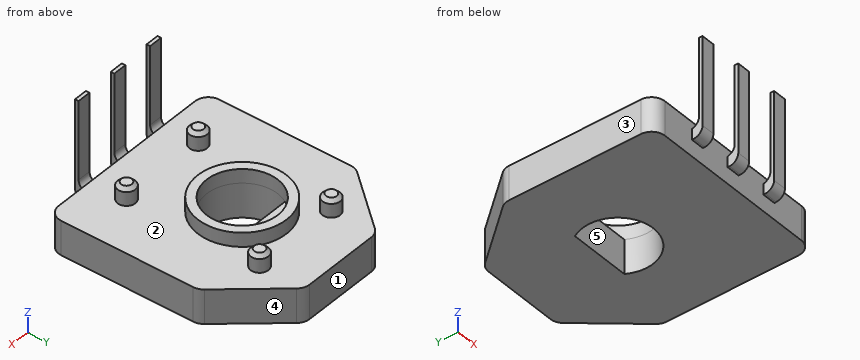
from build123d import *
from build123d.topology import SkipClean

# Parameters (mm, degrees)
BOSS_EXTRUDE1_DEPTH      = 1.93
SKETCH2_R                = 2.5
SKETCH2_R_2              = 2
BOSS_EXTRUDE2_DEPTH      = 0.79
BOSS_EXTRUDE3_DEPTH      = 4.5
BOSS_EXTRUDE3_DEPTH_BACK = 1
SKETCH3_W                = 0.76
SKETCH3_H                = 0.6
FILLET2_R                = 0.75
SKETCH4_W                = 5.74
SKETCH4_H                = 0.4
CUT_EXTRUDE1_DEPTH       = 4.9
FILLET1_R                = 0.5
SKETCH5_R                = 0.5
BOSS_EXTRUDE4_DEPTH      = 0.97
CHAMFER1_SIZE            = 0.2


with BuildPart() as part:
    # Sketch1 → Boss-Extrude1 (new body)
    with BuildSketch(Plane.XY):
        Polygon((5.5, 0), (5.5, -6.5), (-5.5, -6.5), (-5.5, 0), (-5.5, 1.96), (-2.49602332, 5.54), (2.49602332, 5.54), (5.5, 1.96), align=None)
        with BuildLine():
            Line((-1.718566554, 1.023), (1.718566554, 1.023))
            ThreePointArc((1.718566554, 1.023), (0, -2), (-1.718566554, 1.023))
        make_face(mode=Mode.SUBTRACT)
    extrude(amount=BOSS_EXTRUDE1_DEPTH)

    # Sketch2 → Boss-Extrude2 (add)
    with SkipClean():  # the faces are left unmerged after this step: merging them gives an invalid solid
        with BuildSketch(Plane.XY.offset(1.93)):
            with Locations(Location((0, 0, 0), (0, 0, 180))):
                Circle(SKETCH2_R)
            with Locations(Location((0, 0, 0), (0, 0, 149.236204264))):
                Circle(SKETCH2_R_2, mode=Mode.SUBTRACT)
        extrude(amount=BOSS_EXTRUDE2_DEPTH)

    # Sketch3 → Boss-Extrude3 (add, two sides: drawn at the far end of the back side and taken through both)
    with SkipClean():  # the faces are left unmerged after this step: merging them gives an invalid solid
        with BuildSketch(Plane.XY.offset(1.93).offset(-BOSS_EXTRUDE3_DEPTH_BACK)):
            with Locations((0, -6.8)):
                Rectangle(SKETCH3_W, SKETCH3_H)
            with Locations((2.49, -6.8)):
                Rectangle(SKETCH3_W, SKETCH3_H)
            with Locations((-2.49, -6.8)):
                Rectangle(SKETCH3_W, SKETCH3_H)
        extrude(amount=BOSS_EXTRUDE3_DEPTH + BOSS_EXTRUDE3_DEPTH_BACK)

    # Fillet2
    fillet2_edges = [part.edges().sort_by_distance(p)[0] for p in [
        (5.5, -6.5, 0.965),
        (-5.5, -6.5, 0.965),
        (-5.5, 1.96, 0.965),
        (-2.49602332, 5.54, 0.965),
        (2.49602332, 5.54, 0.965),
        (5.5, 1.96, 0.965),
    ]]
    fillet(fillet2_edges, radius=FILLET2_R)

    # Sketch4 → Cut-Extrude1 (cut)
    with SkipClean():  # the faces are left unmerged after this step: merging them gives an invalid solid
        with BuildSketch(Plane.XY.offset(6.43)):
            with Locations((0, -6.7)):
                Rectangle(SKETCH4_W, SKETCH4_H)
        extrude(amount=-CUT_EXTRUDE1_DEPTH, mode=Mode.SUBTRACT)

    # Fillet1
    # the kernel refuses this fillet: 0.5 mm, written as the material it adds along each edge
    with BuildSketch(Plane(origin=(2.87, -6.9, 1.53), x_dir=(0, 1.0, 1.5715206913564052e-12), z_dir=(-1, 0, 0)), Plane(origin=(0.38, -6.9, 1.53), x_dir=(0, 1.0, 1.5715206913564052e-12), z_dir=(-1, 0, 0)), Plane(origin=(-2.11, -6.9, 1.53), x_dir=(0, 1.0, 1.5715206913564052e-12), z_dir=(-1, 0, 0))) as fillet1_piece_1:
        with BuildLine():
            CenterArc((0.5, -0.489897949), FILLET1_R, 101.536959033, 78.463040967)
            Line((0, -0.489897949), (0, 0))
            Line((0, 0), (0.4, 0))
        make_face()
    extrude(amount=0.76)
    # the kernel refuses this fillet: 0.5 mm, written as the material it takes off along each edge
    with BuildSketch(Plane(origin=(0.86, -7.1, 0.93), x_dir=(0, 1, 0), z_dir=(1, 0, 0)), Plane(origin=(-4.12, -7.1, 0.93), x_dir=(0, 1, 0), z_dir=(1, 0, 0))) as fillet1_2_piece_1:
        with BuildLine():
            CenterArc((FILLET1_R, FILLET1_R), FILLET1_R, 180, 90)
            Line((0, FILLET1_R), (0, 0))
            Line((0, 0), (FILLET1_R, 0))
        make_face()
    extrude(amount=3.26, mode=Mode.SUBTRACT)
    with BuildSketch(Plane(origin=(1.63, -7.1, 0.93), x_dir=(0, 1, 0), z_dir=(-1, 0, 0))) as fillet1_2_piece_2:
        with BuildLine():
            CenterArc((FILLET1_R, -FILLET1_R), FILLET1_R, 90, 90)
            Line((0, -FILLET1_R), (0, 0))
            Line((0, 0), (FILLET1_R, 0))
        make_face()
    extrude(amount=3.26, mode=Mode.SUBTRACT)

    # Sketch5 → Boss-Extrude4 (add)
    with BuildSketch(Plane.XY.offset(1.93)):
        with Locations(Location((-2.5, -4.5, 0), (0, 0, 180))):
            Circle(SKETCH5_R)
        with Locations(Location((2.5, -4.5, 0), (0, 0, 180))):
            Circle(SKETCH5_R)
        with Locations(Location((2.5, 3, 0), (0, 0, 180))):
            Circle(SKETCH5_R)
        with Locations(Location((-2.5, 3, 0), (0, 0, 180))):
            Circle(SKETCH5_R)
    extrude(amount=BOSS_EXTRUDE4_DEPTH)

    # Chamfer1
    chamfer1_edges = [part.edges().sort_by_distance(p)[0] for p in [
        (3, -4.5, 2.9),
        (-2, -4.5, 2.9),
        (3, 3, 2.9),
        (-2, 3, 2.9),
    ]]
    chamfer(chamfer1_edges, length=CHAMFER1_SIZE)


solid = part.part
Input: part model. Units: mm. Frame: model coordinates. Face numbers are marked on the shaded views. A direction names the side the tool comes from. Give positions to 0.01 mm unless a question says otherwise; leave off trailing zeros. Write each loop counter-clockwise with the first axis right and the second up, starting at its lowest first coordinate (ties: lowest second). Pieces come first, ordered by that corner, then holes.
Q1. Section B-B, the plane z = 4. Output: boundary loops of the cut face in (x, y), plus the area to 3 significant figures.
Q2. Material intervals for probe 1 along Y at (x, z) = (0, 2.3); probe 2 along X at (y, z) = (0, 1.4); probe 3 along Z at (x, y) = (1.5, 1.75), sorted ascending.
Q3. Set-up query: the marked faces 1 and 2. Return all of +Z, -Z, +X, -X, +Y, -Y with unobstructed straight access to the full face (end or side cutting, diameter ignored); none if empty.
Q4. Section C-C, the plane x = 0. Output: boundary loops of the cut face in (y, z), plus the area to 3 significant figures.
Q5. Section A-A, the plane z = 2.5. State how many separate pieces and enclosed holes the cut face has, plus the area to 3 significant figures.
Q6. First-contact query: P1, Ø4, axis at x = -2.5, y = 1, coming from the +Z side; P2, Ø5.5, axis at x = -2, y = -1, coming from the +Z side; P3, Ø2, axis at x = 4, z = 2, coming from the +Y side. Flat tips, straight axial feed; report the tip coordinate or a pass-through.
Q7. Section D-D, the plane y = -1.75. Output: boundary loops of the cut face in (x, z), plus the area to 3 significant figures.
Q8. Pull-direction query (Y, two-part tool) for the marked faces 3, 4 and 5; classes: pulls with the +Y half, pulls with the -Y half, needs draft (parallel to the pull), parting line crosses it, or undercut.
Filled in:
1. outline: (-2.87, -7.1) - (-2.11, -7.1) - (-2.11, -6.9) - (-2.87, -6.9) - close; (-0.38, -7.1) - (0.38, -7.1) - (0.38, -6.9) - (-0.38, -6.9) - close; (2.11, -7.1) - (2.87, -7.1) - (2.87, -6.9) - (2.11, -6.9) - close
1. area: 0.456 mm2
2. probe 1: y = -7.1 to -6.9, -2.5 to -2, 2 to 2.5
2. probe 2: x = -5.5 to -2, 2 to 5.5
2. probe 3: z = 0 to 2.72
3. face 1: +Z, -Z, +X, -X, +Y
3. face 2: +Z
4. outline: (-7.1, 1.43) arc R0.5 ccw to (-6.6, 0.93) - (-6.5, 0.93) - (-6.5, 0) - (-2, 0) - (-2, 2.72) - (-2.5, 2.72) - (-2.5, 1.93) - (-6.5, 1.93) - (-6.5, 1.53) arc R0.5 cw to (-6.9, 2.02) - (-6.9, 6.43) - (-7.1, 6.43) - close; (1.02, 0) - (5.54, 0) - (5.54, 1.93) - (2.5, 1.93) - (2.5, 2.72) - (2, 2.72) - (2, 1.93) - (1.02, 1.93) - close
4. area: 19.5 mm2
5. separate pieces: 8
5. enclosed holes: 1
5. area: 10.7 mm2
6. P1: stops at z = 2.9
6. P2: stops at z = 2.72
6. P3: stops at y = 4.94
7. outline: (-5.5, 0) - (-0.97, 0) - (-0.97, 2.72) - (-1.79, 2.72) - (-1.79, 1.93) - (-5.5, 1.93) - close; (0.97, 0) - (5.5, 0) - (5.5, 1.93) - (1.79, 1.93) - (1.79, 2.72) - (0.97, 2.72) - close
7. area: 18.8 mm2
8. face 3: needs draft
8. face 4: pulls with the +Y half
8. face 5: undercut
